Here's how the part is built. I have some questions about the finished solid (model axes, mm). A direction names the side the tool comes from. Coordinates: 2 decimals unless noted, no trailing zeros. Order: outer loops, then holes, each group sorted by start corner. A loop starts at its lowest first (then second) coordinate and runs counter-clockwise, first axis right, second up. Notation, with made-up numbers: (40, -16) - (56, -16) arc R26 cw to (56, 18) - close; hole circle Ø1 at (84, -8.5). An arc over 180 degrees is marked (long way). Answer as CSV lines item,"result". Start each with the question number.
Item 1: Imagine slicing it at B-B on y = 0. List the corners of the cut face in (x, z) for me.
Item 2: Imagine slicing it at C-C on x = 39.5. List the corners of the cut face in (y, z) for me.
Item 3: I need wall thicknesses on line 1 (Y direction, x = 0, z = 19); line 2 (X direction, y = 8, z = 14.5); line 3 (Y direction, x = 5.5, z = 7.5). Which ranges of each line are inside material? Lowest first, please.
Item 4: I'm going to push flat-ended pins straight in: pin 1 (2.5 mm diameter, centred on y = 6.5, z = 19, fed in from -X); pin 2 (10 mm diameter, centred on x = 38, z = 13, fed in from -Y); pin 3 (12 mm diameter, centred on x = 23.5, z = 18, fed in from +Y). Where does each tip first touch, or does it pass through?
Item 5: On a 3-axis mill with a long thin cutter (end or side, diameter ignored), from which of +Z, -Z, +X, -X, +Y, -Y can I reach the whole of each face in a straight line? I mean faces 1 (the face through (92.3, 5.3, 3.5)), 2 (the face through (68.168, -5.807, 20.056)), 3 (the face through (68.17, 6.04, 19.94)), 4 (the face through (68.168, 5.926, 3.944)). Say none if no direction works.
Item 6: We'd pull the mould along Y, two halves only. Please class faces 5 (the face through (44, -9.863, 12)), 6 (the face through (-2.17, -9.76, 11.83)), 7 (the face through (56, 7, 3)): pulls with the +Y half, pulls with the -Y half, needs draft (parallel to the pull), parting line crosses it, or undercut.
Item 7: Imagine slicing it at D-D on y = 14. List the corners of the cut face in (x, z) for me.
Item 8: Imagine slicing it at A-A on x = 0. List the corners of the cut face in (y, z) for me, and give its area (3 significant figures).
from build123d import *

# Parameters (mm, degrees)
SKETCH1_R           = 10
BOSS_EXTRUDE4_DEPTH = 24
CUT_EXTRUDE1_DEPTH  = 24
SKETCH8_R           = 10
BOSS_EXTRUDE5_DEPTH = 25


with BuildPart() as part:
    # Sketch1 → Boss-Extrude4 (new body)
    with BuildSketch(Plane.XY):
        with BuildLine():
            Line((19.506185094, 9.982444102), (80, 9.982444102))
            Line((80, 9.982444102), (80, -9.863013699))
            Line((80, -9.863013699), (19.591244248, -9.863013699))
            ThreePointArc((19.591244248, -9.863013699), (17.753039843, -10.310408378), (16.326036873, -11.552511416))
            ThreePointArc((16.326036873, -11.552511416), (-19.99990669, -0.061093452), (16.255154245, 11.652036752))
            ThreePointArc((16.255154245, 11.652036752), (17.678841312, 10.424240243), (19.506185094, 9.982444102))
        make_face()
        Circle(SKETCH1_R, mode=Mode.SUBTRACT)
    extrude(amount=BOSS_EXTRUDE4_DEPTH)

    # Sketch7 → Cut-Extrude1 (cut)
    with BuildSketch(Plane(origin=(80, 0, 0), x_dir=(0, 0, -1), z_dir=(1, 0, 0))):
        Polygon((-8, 9.982444102), (0, 9.982444102), (0, 1.982444102), align=None)
        Polygon((-24, 9.982444102), (-16, 9.982444102), (-24, 1.982444102), align=None)
        Polygon((-24, -9.863013699), (-24, -1.863013699), (-16, -9.863013699), align=None)
        Polygon((0, -9.863013699), (0, -1.863013699), (-8, -9.863013699), align=None)
    extrude(amount=-CUT_EXTRUDE1_DEPTH, mode=Mode.SUBTRACT)

    # Sketch8 → Boss-Extrude5 (add)
    with BuildSketch(Plane(origin=(80, 0, 0), x_dir=(0, 0, -1), z_dir=(1, 0, 0))):
        with Locations(Location((-12, 0.029857601, 0), (0, 0, 214.226665148))):
            Circle(SKETCH8_R)
    extrude(amount=BOSS_EXTRUDE5_DEPTH)


solid = part.part
Responses:
1,outline,"(-20, 0) - (-10, 0) - (-10, 24) - (-20, 24) - close; (10, 0) - (80, 0) - (80, 2) - (105, 2) - (105, 22) - (80, 22) - (80, 24) - (10, 24) - close"
2,outline,"(-9.86, 0) - (9.98, 0) - (9.98, 24) - (-9.86, 24) - close"
3,line 1,"y = -20 to -10, 10 to 20"
3,line 2,"x = -18.33 to -6, 6 to 105"
3,line 3,"y = -19.23 to -8.35, 8.35 to 19.23"
4,pin 1,"stops at x = -19.3"
4,pin 2,"stops at y = -9.86"
4,pin 3,"stops at y = 10.52"
5,face 1,"+X"
5,face 2,"+Z, -Y"
5,face 3,"+Z, +Y"
5,face 4,"-Z, +Y"
6,face 5,"pulls with the -Y half"
6,face 6,"undercut"
6,face 7,"needs draft"
7,outline,"(-14.28, 0) - (14.28, 0) - (14.28, 24) - (-14.28, 24) - close"
8,outline,"(-20, 0) - (-10, 0) - (-10, 24) - (-20, 24) - close; (10, 0) - (20, 0) - (20, 24) - (10, 24) - close"
8,area,"480 mm^2"
